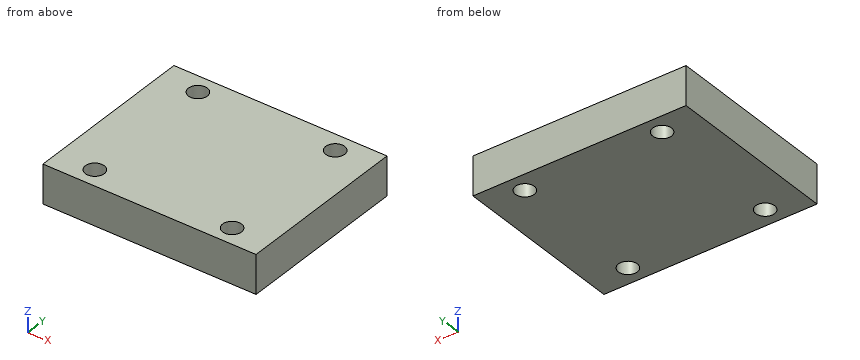
Autodesk Inventor part; units mm, degrees
ref_plane "YZ Plane" through (0, 0, 0) normal (1, 0, 0) x (0, 1, 0)
ref_plane "XZ Plane" through (0, 0, 0) normal (0, 1, 0) x (-1, 0, 0)
ref_plane "XY Plane" through (0, 0, 0) normal (0, 0, 1) x (1, 0, 0)
sketch "Sketch1" plane through (0, 0, 0) normal (0, 0, 1) x (1, 0, 0)
  line L0 (0, 0) -> (57.15, 0)
  line L1 (57.15, 0) -> (57.15, 57.15)
  line L2 (57.15, 57.15) -> (0, 57.15)
  line L3 (0, 57.15) -> (0, 0)
  line L4 (0, 57.15) -> (57.15, 0) construction
  circle A0 centre (28.575, 28.575) radius 31.825 construction
  line L5 (0, 0) -> (57.15, 57.15) construction
  circle A1 centre (6.0713, 51.0787) radius 3.1
  circle A2 centre (6.0713, 6.0713) radius 3.1
  circle A3 centre (51.0787, 6.0713) radius 3.1
  circle A4 centre (51.0787, 51.0787) radius 3.1
  dimension "d2" = 63.65
  dimension "d0" = 57.15
  dimension "d1" = 57.15
  dimension "d3" = 6.2
  dimension "d6" = 360
extrude "Extrusion1" add sketch "Sketch1" along normal blind 12.7
sketch "Sketch2" plane through (0, 0, 12.7) normal (0, 0, 1) x (1, 0, 0)
  line L0 (0, 0) -> (-6.35, 0)
  line L1 (-6.35, 0) -> (-6.35, 57.15)
  line L2 (-6.35, 57.15) -> (0, 57.15)
  line L3 (0, 57.15) -> (0, 0)
  line L4 (57.15, 0) -> (57.15, 57.15)
  line L5 (57.15, 57.15) -> (63.5, 57.15)
  line L6 (63.5, 57.15) -> (63.5, 0)
  line L7 (63.5, 0) -> (57.15, 0)
  line L8 (57.15, 0) -> (57.15, 57.15)
  dimension "d10" = 6.35
  dimension "d11" = 6.35
extrude "Extrusion2" add sketch "Sketch2" against normal up to surface (12.7 mm away)
properties part number "polycarb_back" material "Polycarbonate, Smoke"
Work out the finished part from the listing and answer in its coordinate system (mm). Round coordinates to 2 decimals unless told otherwise and drop trailing zeros. Write each loop counter-clockwise with the first axis right and the second up, starting at its lowest first coordinate (ties: lowest second). Pieces come first, ordered by that corner, then holes.
1) Straight lines are drawn through the part: line 1 (X direction, y = 52.5, z = 1.5); line 2 (X direction, y = 4.5, z = 4.25). For each, find the intervals that lie inside material, in ascending order.
2) A cutting plane is placed at C-C (z = 1). Give the vertices of the cut face in (x, y).
3) A cutting plane is placed at A-A (x = 53). Give the vertices of the cut face in (y, z), plus the area to 3 significant figures.
4) Given pin 1 Ø3.5 at (x, y) = (51.08, 51.08) entering from +Z, flat-ended and moving along its own axis, determine where the tip first touches the part or whether it passes through.
5) A cutting plane is placed at B-B (y = 49). Give the vertices of the cut face in (x, z).
Completed:
1. line 1: x = -6.35 to 3.32, 8.83 to 48.32, 53.83 to 63.5
1. line 2: x = -6.35 to 3.4, 8.74 to 48.41, 53.75 to 63.5
2. outline: (-6.35, 0) - (63.5, 0) - (63.5, 57.15) - (-6.35, 57.15) - close; hole circle Ø6.2 at (6.07, 6.07); hole circle Ø6.2 at (6.07, 51.08); hole circle Ø6.2 at (51.08, 6.07); hole circle Ø6.2 at (51.08, 51.08)
3. outline: (0, 0) - (3.64, 0) - (3.64, 12.7) - (0, 12.7) - close; (8.5, 0) - (48.65, 0) - (48.65, 12.7) - (8.5, 12.7) - close; (53.51, 0) - (57.15, 0) - (57.15, 12.7) - (53.51, 12.7) - close
3. area: 602 mm2
4. pin 1: passes through
5. outline: (-6.35, 0) - (3.77, 0) - (3.77, 12.7) - (-6.35, 12.7) - close; (8.37, 0) - (48.78, 0) - (48.78, 12.7) - (8.37, 12.7) - close; (53.38, 0) - (63.5, 0) - (63.5, 12.7) - (53.38, 12.7) - close
